Autodesk Inventor part; units mm, degrees
ref_plane "作業平面2" through (30, 0, 0) normal (1, 0, 0) x (0, 0, -1)
ref_plane "YZ Plane" through (0, 0, 0) normal (1, 0, 0) x (0, 1, 0)
ref_plane "XZ Plane" through (0, 0, 0) normal (0, 1, 0) x (-1, 0, 0)
sketch "スケッチ3" plane through (0, 0, 0) normal (1, 0, 0) x (0, 1, 0)
  circle A0 centre (436.4013, 3.8245) radius 122.5
  line L0 (299.9013, 146.3245) -> (303.9013, 146.3245)
  line L1 (303.9013, 146.3245) -> (303.9013, -202.8865)
  line L2 (303.9013, -202.8865) -> (299.9013, -202.8865)
  line L3 (299.9013, -202.8865) -> (299.9013, 146.3245)
  line L4 (436.4013, 3.8245) -> (523.0219, 90.445)
  line L5 (436.4013, 3.8245) -> (436.4013, 126.3245)
  line L6 (436.4013, 3.8245) -> (375.1513, 109.9126)
  line L7 (285.9013, 16.0245) -> (238.1013, 16.0245)
  line L8 (238.1013, 16.0245) -> (238.1013, -8.3755)
  line L9 (238.1013, -8.3755) -> (285.9013, -8.3755)
  line L10 (285.9013, -8.3755) -> (285.9013, 16.0245)
  line L11 (285.9013, 10.3245) -> (288.5013, 10.3245)
  line L12 (288.5013, 10.3245) -> (288.5013, -2.6755)
  line L13 (288.5013, -2.6755) -> (285.9013, -2.6755)
  line L14 (285.9013, -2.6755) -> (285.9013, 10.3245)
  line L15 (288.5013, 6.8245) -> (302.9013, 6.8245)
  line L16 (302.9013, 6.8245) -> (302.9013, 0.8245)
  line L17 (302.9013, 0.8245) -> (288.5013, 0.8245)
  line L18 (288.5013, 0.8245) -> (288.5013, 6.8245)
  line L19 (289.9013, 74.154) -> (285.9013, 74.154)
  line L20 (285.9013, 74.154) -> (285.9013, -68.3086)
  line L21 (285.9013, -68.3086) -> (289.9013, -68.3086)
  line L22 (289.9013, -68.3086) -> (289.9013, 74.154)
  line L23 (299.9013, 12.8245) -> (293.9013, 12.8245)
  line L24 (293.9013, 12.8245) -> (293.9013, -5.1755)
  line L25 (293.9013, -5.1755) -> (299.9013, -5.1755)
  line L26 (299.9013, -5.1755) -> (299.9013, 12.8245)
  line L27 (375.1513, 109.9126) -> (303.9013, 109.9126)
  circle A1 centre (-96.0987, 3.8245) radius 600
  line L28 (303.9013, 146.3245) -> (428.795, 146.3245)
  arc A2 (523.0219, 90.445) -> (428.795, 146.3245) centre (439.4013, 56.8245) ccw
  circle A3 centre (-96.0987, 3.8245) radius 400
  circle A4 centre (302.4013, 137.3245) radius 1.5
  circle A5 centre (302.4013, 119.3245) radius 1.5
  line L29 (303.9013, 109.9126) -> (299.9013, 109.9126)
  line L30 (303.9013, 146.3245) -> (318.9013, 146.3245)
  line L31 (318.9013, 146.3245) -> (318.9013, 109.9126)
  line L32 (318.9013, 109.9126) -> (303.9013, 109.9126)
  line L33 (303.9013, 109.9126) -> (303.9013, 146.3245)
  circle A6 centre (311.4013, 131.3245) radius 1.5
  circle A7 centre (311.4013, 116.3245) radius 1.5
  line L34 (328.9013, 146.3245) -> (328.9013, 109.9126)
  circle A8 centre (501.4013, 128.9702) radius 1.7
  circle A9 centre (350.4013, 151.3245) radius 1.7
  circle A10 centre (501.4013, 128.9702) radius 5
  circle A11 centre (350.4013, 151.3245) radius 5
  line L35 (345.4013, 151.3245) -> (345.4013, 146.3245)
  line L36 (355.4013, 151.3245) -> (355.4013, 146.3245)
  circle A12 centre (335.4013, 151.3245) radius 5
  circle A13 centre (335.4013, 151.3245) radius 1.7
  line L37 (328.9013, 146.3245) -> (328.9013, 156.3245)
  line L38 (328.9013, 156.3245) -> (436.4013, 156.3245)
  circle A14 centre (489.2896, 137.8193) radius 5
  circle A15 centre (489.2896, 137.8193) radius 1.7
  circle A16 centre (103.9013, 3.8245) radius 600
  line L39 (523.0219, 90.445) -> (506.0106, 130.908)
  line L40 (436.4013, 156.3245) -> (490.5132, 142.6673)
  line L41 (492.2393, 141.8565) -> (504.351, 133.0074)
  line L42 (485.1551, 140.631) -> (482.1278, 136.1793)
  line L43 (493.4242, 135.0077) -> (490.6655, 130.9509)
  point P0 (0, 0)
  point P1 (303.9013, 128.1185)
  point P2 (497.234, 131.733)
  point P3 (453.1551, 145.8951)
  point P4 (497.1922, 131.669)
  point P5 (463.1906, 143.7544)
  point P6 (497.2988, 131.8284)
  point P7 (497.321, 131.86)
  point P8 (350.4013, 156.3245)
  point P9 (350.4013, 146.3245)
  point P10 (498.1425, 125.1781)
  point P11 (521.9251, 93.054)
  dimension "d65" = 3
  dimension "d66" = 3
  dimension "d67" = 9
  dimension "d68" = 18
  dimension "d69" = 2.5
  dimension "d70" = 2.5
  dimension "d71" = 15
  dimension "d72" = 0
  dimension "d73" = 3
  dimension "d74" = 3
  dimension "d75" = 15
  dimension "d76" = 15
  dimension "d77" = 7.5
  dimension "d78" = 7.5
  dimension "d79" = 10
  dimension "d80" = 3.4
  dimension "d81" = 3.4
  dimension "d82" = 10
  dimension "d83" = 10
  dimension "d84" = 86
  dimension "d85" = 10
  dimension "d86" = 3.4
  dimension "d87" = 15
  dimension "d88" = 10
  dimension "d89" = 3.4
  dimension "d90" = 15
  dimension "d91" = 65
extrude "押し出し4" add sketch "スケッチ3" along normal blind 60 contours A0 A1 A2 L39 | A0 L27 L34 L28 A2 A1
extrude "押し出し5" add sketch "スケッチ3" along normal blind 10 contours A2 A14 A1 | A1 A14 L43 A2 | A14 A1 A15 | A1 A15 A14 | A2 L42 A14 | L35 A11 L28 | A11 | L28 A11 L36
fillet "フィレット2" radius 2 6 edges at (10, 350.4013, 146.3245) (5, 345.4013, 146.3245) (5, 355.4013, 146.3245) (5, 482.1278, 136.1793) (5, 490.6655, 130.9509) (10, 486.4693, 133.6838)
ref_plane "作業平面2" through (30, 0, 0) normal (1, 0, 0) x (0, 0, -1)
mirror "ミラー2" about plane through (30, 0, 0) normal (1, 0, 0) of "押し出し5", "フィレット2"
equation "\"d70\" = d69"
properties part number "hand-grab-v2-3DP-arm-C" material "ABS プラスチック"
The model under review builds one solid part; all positions refer to its coordinate system, in mm. A direction names the side the tool comes from. Give positions to 0.01 mm unless a question says otherwise; leave off trailing zeros. Write each loop counter-clockwise with the first axis right and the second up, starting at its lowest first coordinate (ties: lowest second). Pieces come first, ordered by that corner, then holes.
1. Add section A-A, the plane z = 115. Write out the cut boundary in (x, y).
2. Tool access review of faces 1 (the flat face through (30, 352, 109.913)), 2 (the flat face through (10, 491, 139)), 3 (the flat face through (50, 350.5, 153.3)), 4 (the flat face through (30, 378, 146.324)): name each direction out of +Z, -Z, +X, -X, +Y, -Y from which nothing blocks a thin tool from reaching the whole face with its end or side.
3. Add section C-C, the plane y = 368.5. Write out the cut boundary in (x, z), plus the area to 3 significant figures.
4. Draft analysis for pull direction X (two halves, no side actions). For faces 5 (the flat face through (0, 403, 131)), 6 (the flat face through (50, 490, 140)), 7 (the cylindrical face through (4.93, 490.91, 137.31)), state which applies: +X half, -X half, draft (parallel to the pull), parting line (faces both ways), or undercut.
5. Add section D-D, the plane x = 17.5. Write out the cut boundary in (y, z) (1 decimal).
6. For P1, Ø3.5, axis at x = 6, z = 149.5, coming from the -Y side; P2, Ø3, axis at y = 350.4, z = 151.32, coming from the +X side; P3, Ø6, axis at x = 52, z = 103.5, coming from the -Y side; P4, Ø2.5, axis at x = 57, z = 149.5, coming from the +Y side, all flat-tipped, find the tip position at first contact; note any pin that passes through.
7. Add section B-B, the plane x = 6. Write out the cut boundary in (y, z) (1 decimal).
8. Wall thickness on L1, parallel to Z at x = 50, y = 368; L2, parallel to Y at x = 26, z = 116.5; L3, parallel to Y at x = 51, z = 149: over which ranges is each line inside the solid? List them lowest first.
Worked answers:
1. outline: (0, 328.9) - (60, 328.9) - (60, 384.96) - (0, 384.96) - close; (0, 487.84) - (60, 487.84) - (60, 508.24) - (0, 508.24) - close
2. face 1: -Z, +X, -X, -Y
2. face 2: +Z, +Y
2. face 3: +Z, +Y, -Y
2. face 4: +Z
3. outline: (0, 109.91) - (60, 109.91) - (60, 146.32) - (0, 146.32) - close
3. area: 2,180 mm2
4. face 5: -X half
4. face 6: undercut
4. face 7: draft
5. outline: (328.9, 109.9) - (375.2, 109.9) arc R122.5 cw to (523, 90.4) - (521.9, 93.1) arc R90.1 ccw to (428.8, 146.3) - (328.9, 146.3) - close
6. P1: stops at y = 345.32
6. P2: passes through
6. P3: stops at y = 503.21
6. P4: stops at y = 355.4
7. outline: (328.9, 109.9) - (375.2, 109.9) arc R122.5 cw to (523, 90.4) - (521.9, 93.1) arc R90.1 ccw to (492.3, 129.8) arc R2 cw to (491.8, 132.6) - (493.4, 135) arc R5 ccw to (485.2, 140.6) - (483.1, 137.7) arc R2 cw to (480.6, 137) arc R90.1 ccw to (428.8, 146.3) - (357.4, 146.3) arc R2 cw to (355.4, 148.3) - (355.4, 151.3) arc R5 ccw to (345.4, 151.3) - (345.4, 148.3) arc R2 cw to (343.4, 146.3) - (328.9, 146.3) - close; hole circle Ø3.4 at (350.4, 151.3); hole circle Ø3.4 at (489.3, 137.8)
8. L1: z = 109.91 to 146.32
8. L2: y = 328.9 to 388.33, 484.47 to 506.94
8. L3: y = 345.4 to 355.4
